The listing builds one solid part. Answer for the finished solid, in the listing's coordinates (mm). A direction names the side the tool comes from. Coordinates: 2 decimals unless noted, no trailing zeros. Loops run counter-clockwise (first coordinate to the right, second up) from the corner with the lowest first, then second, coordinate; pieces in that order, holes last. Notation, with made-up numbers: (63, -35) -> (113, -35) arc R24 cw to (113, -20) -> close; hole circle Ø4 at (-34.75, 54.5). An arc over 180 degrees is marked (long way). Answer in a Markdown table with one row per item.
```python
from build123d import *

# Parameters (mm, degrees)
F1_DEPTH = 10
F2_R     = 2
F3_DEPTH = 23.001
F5_DEPTH = 15.001
F6_DEPTH = 15
F7_R     = 1.3
F8_DEPTH = 68.901


with BuildPart() as f1:
    # F0 (on Front) → F1 (new body, symmetric)
    with BuildSketch(Plane.XZ):
        Polygon((32.5, 0), (0, 0), (0, -2.5), (30, -2.5), (30, -10.5), (66.4, -10.5), (66.4, -23), (68.9, -23), (68.9, -8), (32.5, -8), align=None)
    extrude(amount=F1_DEPTH, both=True)

    # F2 (on Top) → F3 (cut, through all)
    with BuildSketch(Plane.XY):
        with Locations((41.5, 0)):
            Circle(F2_R)
    extrude(amount=-F3_DEPTH, mode=Mode.SUBTRACT)

    # F4 (on face) → F5 (cut, through all)
    with BuildSketch(Plane.XY.offset(-8)):
        Polygon((70.9, 10), (68.9, 10), (68.9, 0), (68.9, -10), (70.9, -10), align=None)
        with BuildLine():
            Line((68.9, -10), (68.9, 0))
            ThreePointArc((68.9, 0), (68.71737, -5.013288), (68.170448, -10))
            Line((68.170448, -10), (68.9, -10))
        make_face()
        with BuildLine():
            Line((68.9, 10), (68.170448, 10))
            ThreePointArc((68.170448, 10), (68.71737, 5.013288), (68.9, 0))
            Line((68.9, 0), (68.9, 10))
        make_face()
    extrude(amount=-F5_DEPTH, mode=Mode.SUBTRACT)

    # F4 (on face) → F6 (join, through all)
    with BuildSketch(Plane.XY.offset(-8)):
        with BuildLine():
            Line((68.170448, 10), (65.642669, 10))
            ThreePointArc((65.642669, 10), (66.4, 0), (65.642669, -10))
            Line((65.642669, -10), (68.170448, -10))
            ThreePointArc((68.170448, -10), (68.71737, -5.013288), (68.9, 0))
            ThreePointArc((68.9, 0), (68.71737, 5.013288), (68.170448, 10))
        make_face()
    extrude(amount=-F6_DEPTH)

    # F7 (on Right) → F8 (cut, through all)
    with BuildSketch(Plane.YZ):
        with Locations((0, -15)):
            Circle(F7_R)
    extrude(amount=F8_DEPTH, mode=Mode.SUBTRACT)

    # F9: F1 across plane


with BuildPart() as f1_1:
    add(f1.part)
    add(f1.part.mirror(Plane.YZ))


solid = f1_1.part
```
Item 1: Determine the mould class of faces 1 (the face through (15, -10, -2)), 2 (the face through (0, 0, 0)), 3 (the face through (-39.502, 0.088, -9.232)) for opening direction Y: +Y half, -Y half, draft (parallel to the pull), parting line (faces both ways), or undercut.
Findings below:
| item | result |
|---|---|
| face 1 | -Y half |
| face 2 | draft |
| face 3 | undercut |
Item 2: A cutting plane is placed at D-D, the plane z = -15. Determine the outline of the cut face in (x, y).
Findings below:
| item | result |
|---|---|
| outline | (-68.89, -1.3) arc R68.9 ccw to (-68.17, -10) -> (-65.64, -10) arc R66.4 cw to (-66.39, -1.3) -> close; (-68.89, 1.3) -> (-66.39, 1.3) arc R66.4 cw to (-65.64, 10) -> (-68.17, 10) arc R68.9 ccw to start; (65.64, -10) -> (68.17, -10) arc R68.9 ccw to (68.89, -1.3) -> (66.39, -1.3) arc R66.4 cw to start; (65.64, 10) arc R66.4 cw to (66.39, 1.3) -> (68.89, 1.3) arc R68.9 ccw to (68.17, 10) -> close |
Item 3: A tool of negligible diameter and unlimited length cuts with its end or side. For faces 4 (the face through (51, 0, -8)), 5 (the face through (-66.4, 0.1, -16.7)), 6 (the face through (-51, 0, -8)), from which of +Z, -Z, +X, -X, +Y, -Y can it reach the whole face along a straight path? Write none if from no direction.
Findings below:
| item | result |
|---|---|
| face 4 | +Z, +X, +Y, -Y |
| face 5 | -Z |
| face 6 | +Z, -X, +Y, -Y |
Item 4: A cutting plane is placed at A-A, the plane x = 41.5. Determine the outline of the cut face in (y, z), plus the area to 3 significant figures.
Findings below:
| item | result |
|---|---|
| outline | (-10, -10.5) -> (-2, -10.5) -> (-2, -8) -> (-10, -8) -> close; (2, -10.5) -> (10, -10.5) -> (10, -8) -> (2, -8) -> close |
| area | 40.0 mm2 |
Item 5: A cutting plane is placed at C-C, the plane y = -7. Determine the outline of the cut face in (x, z).
Findings below:
| item | result |
|---|---|
| outline | (-68.54, -23) -> (-66.03, -23) -> (-66.03, -10.5) -> (-30, -10.5) -> (-30, -2.5) -> (30, -2.5) -> (30, -10.5) -> (66.03, -10.5) -> (66.03, -23) -> (68.54, -23) -> (68.54, -8) -> (32.5, -8) -> (32.5, 0) -> (-32.5, 0) -> (-32.5, -8) -> (-68.54, -8) -> close |
Item 6: Flat-ended cylindrical pins translate along their axes: pin 1 Ø4 at (x, y) = (-36, 1.5) entering from +Z; pin 2 Ø4 at (y, z) = (1, -3) entering from +X; pin 3 Ø4 at (y, z) = (-2, -7) entering from -X. Find the tip coordinate at first contact, or state that the pin passes through.
Findings below:
| item | result |
|---|---|
| pin 1 | stops at z = -8 |
| pin 2 | stops at x = 32.5 |
| pin 3 | stops at x = -68.9 |
Item 7: Find the intervals of material crossed by probe 1 along X at (y, z) = (0.25, -10); probe 2 along X at (y, z) = (6.25, -7.5); probe 3 along Y at (x, z) = (41.5, -9.9), in increasing order.
Findings below:
| item | result |
|---|---|
| probe 1 | x = -68.9 to -43.48, -39.52 to -30, 30 to 39.52, 43.48 to 68.9 |
| probe 2 | x = -32.5 to -30, 30 to 32.5 |
| probe 3 | y = -10 to -2, 2 to 10 |
Item 8: A cutting plane is placed at B-B, the plane z = -6. Determine the outline of the cut face in (x, y).
Findings below:
| item | result |
|---|---|
| outline | (-32.5, -10) -> (-30, -10) -> (-30, 10) -> (-32.5, 10) -> close; (30, -10) -> (32.5, -10) -> (32.5, 10) -> (30, 10) -> close |
